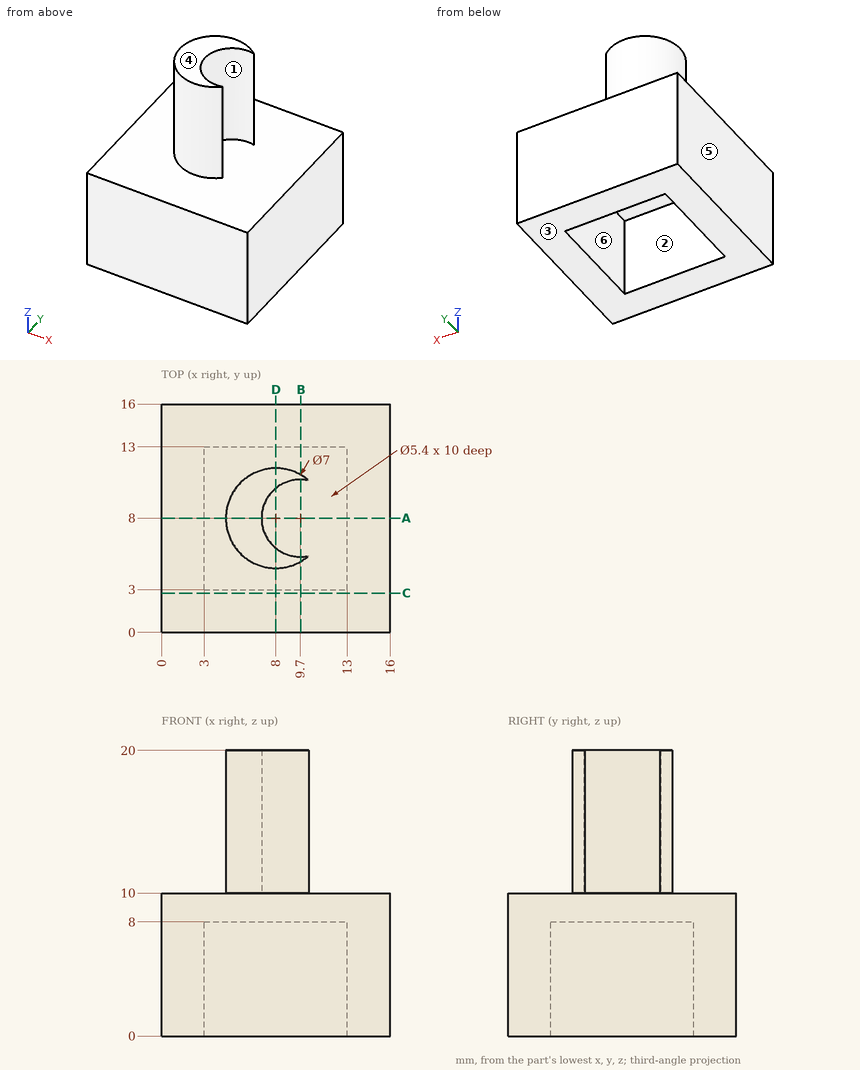
Source: three-view drawing plus pictorial views. Frame: mm from the lowest corner of the part. A direction names the side the tool comes from. Round coordinates to 2 decimals unless told otherwise and drop trailing zeros. Loops run counter-clockwise (first coordinate to the right, second up) from the corner with the lowest first, then second, coordinate; pieces in that order, holes last. Notation, with made-up numbers: (59.25, 39.5) - (77.25, 39.5) arc R32 cw to (77.25, 66.5) - close; hole circle Ø8 at (-8.5, 37.5). An arc over 180 degrees is marked (long way). Write item = value, one per line. Start each with the question number.
Item 1: Section query B-B on x = 9.75. Output: boundary loops of the cut face in (y, z), plus the area to 3 significant figures.
Item 2: Material intervals for line 1 (X direction, y = 4, z = 1.75); line 2 (Z direction, x = 0.5, y = 4.25), sorted ascending.
Item 3: First-contact query: pin 1 Ø1 at (x, y) = (2, 4) entering from +Z; pin 2 Ø5 at (x, y) = (6, 6.5) entering from -Z. Flat tips, straight axial feed; report the tip coordinate or a pass-through.
Item 4: Mould query, pull axis X, two halves, no side actions, for the marked faces 4, 5 and 6. Classes: released by +X, released by -X, zero draft, split by the parting line, or undercut.
Item 5: Section query C-C on y = 2.75. Output: boundary loops of the cut face in (x, z), plus the area to 3 significant figures.
Item 6: Section query A-A on y = 8. Output: boundary loops of the cut face in (x, z), plus the area to 3 significant figures.
Item 7: Section query D-D on x = 8. Output: boundary loops of the cut face in (y, z), plus the area to 3 significant figures.
Item 8: Reachability of the marked faces 1, 2 and 3 from +Z, -Z, +X, -X, +Y, -Y: full face, straight path, thin tool, end or side. Return the list, or none.
Results list:
q1.outline = (0, 0) - (3, 0) - (3, 8) - (13, 8) - (13, 0) - (16, 0) - (16, 10) - (11.03, 10) - (11.03, 20) - (10.7, 20) - (10.7, 10) - (5.3, 10) - (5.3, 20) - (4.97, 20) - (4.97, 10) - (0, 10) - close
q1.area = 86.6 mm²
q2.line_1 = 0 to 3, 13 to 16
q2.line_2 = 0 to 10
q3.pin_1 = 10
q3.pin_2 = 8
q4.face_4 = zero draft
q4.face_5 = released by -X
q4.face_6 = undercut
q5.outline = (0, 0) - (16, 0) - (16, 10) - (0, 10) - close
q5.area = 160 mm²
q6.outline = (0, 0) - (3, 0) - (3, 8) - (13, 8) - (13, 0) - (16, 0) - (16, 10) - (7, 10) - (7, 20) - (4.5, 20) - (4.5, 10) - (0, 10) - close
q6.area = 105 mm²
q7.outline = (0, 0) - (3, 0) - (3, 8) - (13, 8) - (13, 0) - (16, 0) - (16, 10) - (11.5, 10) - (11.5, 20) - (10.1, 20) - (10.1, 10) - (5.9, 10) - (5.9, 20) - (4.5, 20) - (4.5, 10) - (0, 10) - close
q7.area = 108 mm²
q8.face_1 = +Z
q8.face_2 = -Z
q8.face_3 = -Z, +X, -X, +Y, -Y
